Geometry: see drawing. Coordinates: mm, zero at the bounding-box minimum. A direction names the side the tool comes from. Round coordinates to 2 decimals unless told otherwise and drop trailing zeros. Order: outer loops, then holes, each group sorted by start corner. A loop starts at its lowest first (then second) coordinate and runs counter-clockwise, first axis right, second up. Notation, with made-up numbers: (22, 27.25) -> (34, 27.25) arc R24 ccw to (34, 48.25) -> close; hole circle Ø7 at (74, 64.25). An arc over 180 degrees is marked (long way). Put each result on its own line as item: value.
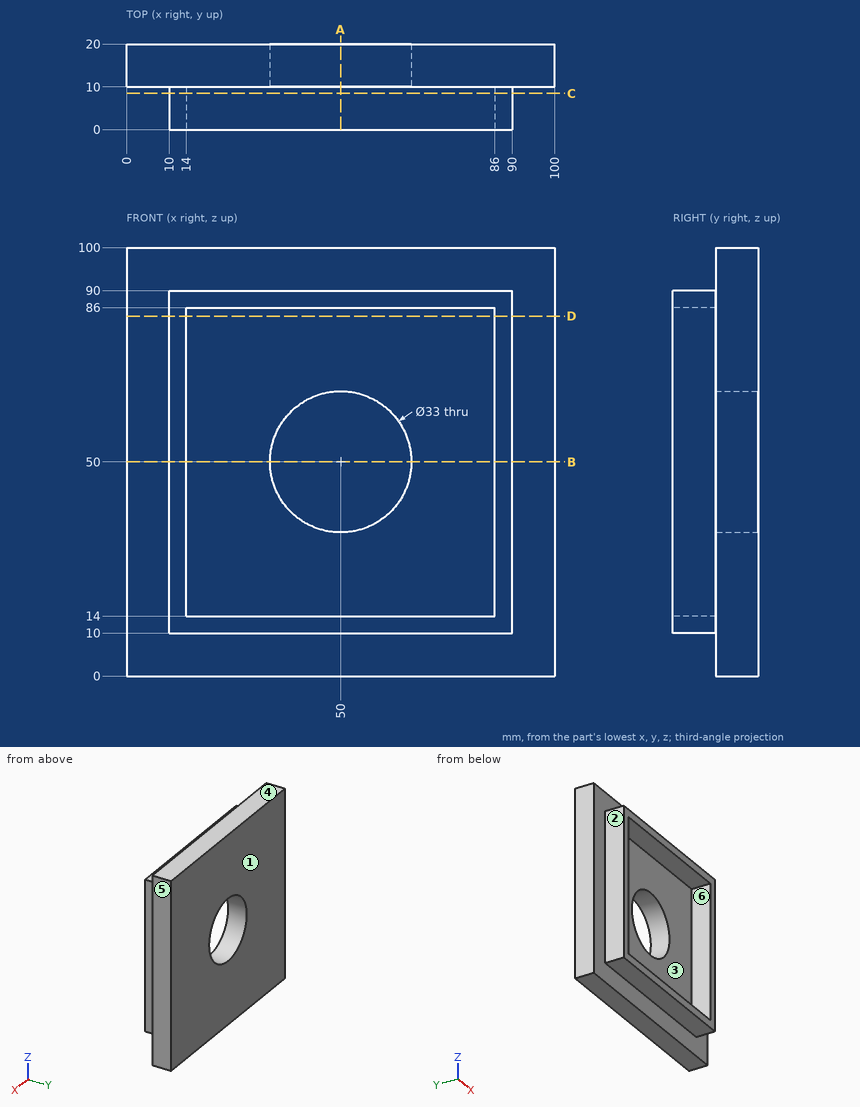
1. Cut plane B-B on z = 50. Return loops of the section in (x, y).
Ans:
outline: (0, 10) -> (10, 10) -> (10, 0) -> (14, 0) -> (14, 10) -> (33.5, 10) -> (33.5, 20) -> (0, 20) -> close; (66.5, 10) -> (86, 10) -> (86, 0) -> (90, 0) -> (90, 10) -> (100, 10) -> (100, 20) -> (66.5, 20) -> close
2. Cut plane C-C on y = 8.5. Return loops of the section in (x, z).
Ans:
outline: (10, 10) -> (90, 10) -> (90, 90) -> (10, 90) -> close; hole (14, 14) -> (86, 14) -> (86, 86) -> (14, 86) -> close
3. Cut plane D-D on z = 84. Return loops of the section in (x, y), and give its area (3 significant figures).
Ans:
outline: (0, 10) -> (10, 10) -> (10, 0) -> (14, 0) -> (14, 10) -> (86, 10) -> (86, 0) -> (90, 0) -> (90, 10) -> (100, 10) -> (100, 20) -> (0, 20) -> close
area: 1,080 mm²
4. Set-up query: the marked faces 1, 2 and 3. Return all of +Z, -Z, +X, -X, +Y, -Y with unobstructed straight access to the full face (end or side cutting, diameter ignored); none if empty.
Ans:
face 1: +Z, -Z, +X, -X, +Y
face 2: +Z, -Z, -X, -Y
face 3: -Y
5. Material intervals for probe 1 along X at (y, z) = (9.5, 73.5); probe 2 along X at (y, z) = (13.5, 50), sorted ascending.
Ans:
probe 1: 10 to 14, 86 to 90
probe 2: 0 to 33.5, 66.5 to 100
6. Draft query along Z for the marked faces 4, 5 and 6. Return one class per face: +Z half, -Z half, draft (parallel to the pull), parting line (faces both ways), or undercut.
Ans:
face 4: +Z half
face 5: draft
face 6: undercut
7. Contact query for flat-ended pins moving along their axis: P1, Ø3, axis at x = 46, y = 3, coming from the +Z side; P2, Ø5, axis at x = 69.5, y = 3, coming from the -Z side; P3, Ø3, axis at y = 7, z = 59, coming from the -X side. Output: stop coordinate, or through.
Ans:
P1: z = 90
P2: z = 10
P3: x = 10
8. Cut plane A-A on x = 50. Return loops of the section in (y, z), and give its area (3 significant figures).
Ans:
outline: (0, 10) -> (10, 10) -> (10, 0) -> (20, 0) -> (20, 33.5) -> (10, 33.5) -> (10, 14) -> (0, 14) -> close; (0, 86) -> (10, 86) -> (10, 66.5) -> (20, 66.5) -> (20, 100) -> (10, 100) -> (10, 90) -> (0, 90) -> close
area: 750 mm²
